from build123d import *

# Parameters (mm, degrees)
F0_W     = 16.002
F0_H     = 32.004
F1_DEPTH = 5.0038
F2_R     = 2.3495
F3_DEPTH = 1.8542
F4_SIZE  = 0.254


with BuildPart() as f1:
    # F0 (on Top) → F1 (new body)
    with BuildSketch(Plane.XY):
        with Locations((-8.001, 16.002)):
            Rectangle(F0_W, F0_H)
    extrude(amount=F1_DEPTH)

    # F2 (on face) → F3 (join)
    with BuildSketch(Plane.XY.offset(5.0038)):
        with Locations((-12.0904, 3.9116)):
            Circle(F2_R)
        with Locations((-11.93851, 11.911158)):
            Circle(F2_R)
        with Locations((-11.634729, 27.910274)):
            Circle(F2_R)
        with Locations((-4.0894, 3.9116)):
            Circle(F2_R)
        with Locations((-3.93751, 11.911158)):
            Circle(F2_R)
        with Locations((-3.785619, 19.910716)):
            Circle(F2_R)
        with Locations((-11.786619, 19.910716)):
            Circle(F2_R)
        with Locations((-3.633729, 27.910274)):
            Circle(F2_R)
    extrude(amount=F3_DEPTH)

    # F4
    f4_edges = [f1.edges().sort_by_distance(p)[0] for p in [
        (-14.4399, 3.9116, 6.858),
        (-14.28801, 11.911158, 6.858),
        (-14.136119, 19.910716, 6.858),
        (-13.984229, 27.910274, 6.858),
        (-5.983229, 27.910274, 6.858),
        (-6.135119, 19.910716, 6.858),
        (-6.28701, 11.911158, 6.858),
        (-6.4389, 3.9116, 6.858),
    ]]
    chamfer(f4_edges, length=F4_SIZE)


solid = f1.part
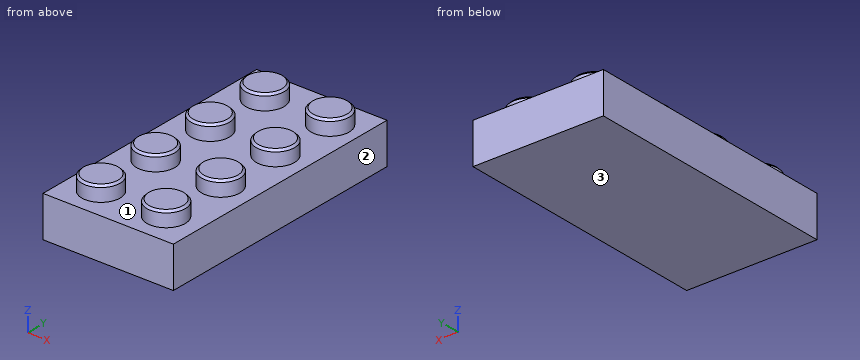
Check sheet for the modelled part. Datum: model origin and axes. Units: mm. Face numbers are marked on the shaded views. Round coordinates to 2 decimals unless told otherwise and drop trailing zeros. Loops run counter-clockwise (first coordinate to the right, second up) from the corner with the lowest first, then second, coordinate; pieces in that order, holes last.
1. Mould release check, pull along X, two halves, no side actions. Record for the marked faces 1, 2 and 3: released by +X, released by -X, zero draft, split by the parting line, or undercut.
2. Sectioned sample at B-B on y = 23. Record the boundary of the cut face in (x, z), and give its area (3 significant figures).
3. Scan lines: probe 1 along Y at (x, z) = (-3.25, 5.5); probe 2 along Z at (x, y) = (-5.75, 13.5); probe 3 along X at (y, z) = (3, 6.5). Record each from-to range of solid material in increasing order.
4. Sectioned sample at C-C on x = -8.5. Record the boundary of the cut face in (y, z).
5. Gauge pin test, flat end, axial feed: pin 1 Ø8 at (x, y) = (-7.5, 11.5) entering from +Z. Record the tip position at first contact, or that the pin passes through.
6. Sectioned sample at A-A on z = 6.25. Record the boundary of the cut face in (x, y).
Recorded:
1. face 1: undercut
1. face 2: released by +X
1. face 3: zero draft
2. outline: (-16, 0) - (0, 0) - (0, 5) - (-16, 5) - close
2. area: 80.1 mm2
3. probe 1: y = 1.72 to 6.11, 9.66 to 14.16, 17.62 to 22.2, 25.59 to 30.23
3. probe 2: z = 0 to 5
3. probe 3: x = -14.26 to -9.92, -6.25 to -1.92
4. outline: (0, 0) - (32, 0) - (32, 5) - (0, 5) - close
5. pin 1: stops at z = 6.86
6. outline: circle Ø4.7 at (-12.09, 3.91); circle Ø4.7 at (-11.94, 11.91); circle Ø4.7 at (-11.79, 19.91); circle Ø4.7 at (-11.63, 27.91); circle Ø4.7 at (-4.09, 3.91); circle Ø4.7 at (-3.94, 11.91); circle Ø4.7 at (-3.79, 19.91); circle Ø4.7 at (-3.63, 27.91)
